from build123d import *

# Parameters (mm, degrees)
BOSS_EXTRUDE1_DEPTH = 1.6
SKETCH4_R           = 1.5
CUT_EXTRUDE1_DEPTH  = 1.6
SKETCH5_R           = 1.5
CUT_EXTRUDE2_DEPTH  = 1.6
SKETCH6_W           = 36.5
SKETCH6_H           = 3
CUT_EXTRUDE3_DEPTH  = 1.6
CUT_EXTRUDE4_DEPTH  = 1.6
CUT_EXTRUDE5_DEPTH  = 1.6
BOSS_EXTRUDE3_START = 1.6
SKETCH9_W           = 81.8
SKETCH9_H           = 2
BOSS_EXTRUDE3_DEPTH = 1


with BuildPart() as part:
    # Sketch2 → Boss-Extrude1 (new body)
    with BuildSketch(Plane.XY):
        Polygon((50, -51.75), (50, 4.25), (33.5, 51.75), (-33.5, 51.75), (-50, 4.25), (-50, -51.75), align=None)
    extrude(amount=BOSS_EXTRUDE1_DEPTH)

    # Sketch4 → Cut-Extrude1 (cut)
    with BuildSketch(Plane.XY.offset(1.6)):
        with Locations((-45.5, -48.75)):
            Circle(SKETCH4_R)
        with Locations((-45.5, -26.75)):
            Circle(SKETCH4_R)
        with Locations(Location((45.5, -26.75, 0), (0, 0, 180))):
            Circle(SKETCH4_R)
        with Locations(Location((45.5, -48.75, 0), (0, 0, 180))):
            Circle(SKETCH4_R)
    extrude(amount=-CUT_EXTRUDE1_DEPTH, mode=Mode.SUBTRACT)

    # Sketch5 → Cut-Extrude2 (cut)
    with BuildSketch(Plane.XY.offset(1.6)):
        with Locations((-18.25, 39.25)):
            Circle(SKETCH5_R)
        with Locations(Location((18.25, 39.25, 0), (0, 0, 180))):
            Circle(SKETCH5_R)
    extrude(amount=-CUT_EXTRUDE2_DEPTH, mode=Mode.SUBTRACT)

    # Sketch6 → Cut-Extrude3 (cut)
    with BuildSketch(Plane.XY.offset(1.6)):
        with Locations((0, 39.25)):
            Rectangle(SKETCH6_W, SKETCH6_H)
    extrude(amount=-CUT_EXTRUDE3_DEPTH, mode=Mode.SUBTRACT)

    # Sketch7 → Cut-Extrude4 (cut)
    with BuildSketch(Plane.XY):
        with BuildLine():
            Line((-33.55, -11.75), (33.55, -11.75))
            ThreePointArc((33.55, -11.75), (34.575304833, -11.325304833), (35, -10.3))
            Line((35, -10.3), (35, -10.2))
            ThreePointArc((35, -10.2), (34.575304833, -9.174695167), (33.55, -8.75))
            Line((33.55, -8.75), (-33.55, -8.75))
            ThreePointArc((-33.55, -8.75), (-34.575304833, -9.174695167), (-35, -10.2))
            Line((-35, -10.2), (-35, -10.3))
            ThreePointArc((-35, -10.3), (-34.575304833, -11.325304833), (-33.55, -11.75))
        make_face()
    extrude(amount=CUT_EXTRUDE4_DEPTH, mode=Mode.SUBTRACT)

    # Sketch8 → Cut-Extrude5 (cut)
    with BuildSketch(Plane.XY):
        with BuildLine():
            Line((-33.55, 11.25), (33.55, 11.25))
            ThreePointArc((33.55, 11.25), (34.575304833, 11.674695167), (35, 12.7))
            Line((35, 12.7), (35, 12.8))
            ThreePointArc((35, 12.8), (34.575304833, 13.825304833), (33.55, 14.25))
            Line((33.55, 14.25), (-33.55, 14.25))
            ThreePointArc((-33.55, 14.25), (-34.575304833, 13.825304833), (-35, 12.8))
            Line((-35, 12.8), (-35, 12.7))
            ThreePointArc((-35, 12.7), (-34.575304833, 11.674695167), (-33.55, 11.25))
        make_face()
    extrude(amount=CUT_EXTRUDE5_DEPTH, mode=Mode.SUBTRACT)

    # Sketch9 → Boss-Extrude3 (add)
    with BuildSketch(Plane.XY.offset(BOSS_EXTRUDE3_START)):
        Polygon((50, -23.75), (50, 4.25), (33.5, 51.75), (-33.5, 51.75), (-50, 4.25), (-50, -23.75), (-48, -23.75), (-48, 3.91252214), (-32.077507691, 49.75), (32.077507691, 49.75), (48, 3.91252214), (48, -23.75), align=None)
        with Locations((0, -50.75)):
            Rectangle(SKETCH9_W, SKETCH9_H)
    extrude(amount=BOSS_EXTRUDE3_DEPTH)


solid = part.part
For this review, take the finished solid that the model builds, in its own axes (mm). A direction names the side the tool comes from. Coordinates: 2 decimals unless noted, no trailing zeros. Write each loop counter-clockwise with the first axis right and the second up, starting at its lowest first coordinate (ties: lowest second). Pieces come first, ordered by that corner, then holes. Notation, with made-up numbers: (4, 25) -> (40, 25) arc R18 ccw to (40, 41) -> close; hole circle Ø11 at (-5, -27.75). An arc over 180 degrees is marked (long way). Write each question's results on one line, items separated by ' | '. Start each with the question number.
1) Consider section C-C (y = 26.5). Write out the cut boundary in (x, z), plus the area to 3 significant figures.
2) Insertion check: pin 1 (6 mm diameter, centred on x = -32, y = 36, fed in from +Z); pin 2 (2.5 mm diameter, centred on x = -45.5, y = -48.75, fed in from +Z). Each pin has a flat end and moves straight along its axis. Give the tip position at first contact, or say it passes through.
3) Consider section D-D (x = 45.5). Write out the cut boundary in (y, z).
4) Consider section A-A (z = 0.7). Give the number of separate pieces and of enclosed holes in the cut face, plus the area to 4 significant figures.
5) Consider section B-B (x = -24). Write out the cut boundary in (y, z).
6) Wall thickness on L1, parallel to Y at x = 16.5, z = 0.85; L2, parallel to Y at x = -23, z = 2.2; L3, parallel to Z at x = 20.5, y = 11: over which ranges is each line inside the solid? List them lowest first. Write a range as [from, to].
7) The part is to be moulded in two halves that separate along X. For faces 1 (the face through (0, 51.75, 1)), 2 (the face through (-41.634, 28.332, 1.282)), 3 (the face through (50, -24, 1)), 4 (the face through (46.69, -47.84, 0.81)), say which applies: +X half, -X half, draft (parallel to the pull), parting line (faces both ways), or undercut.
8) For faces 5 (the face through (-40.15, 26.51, 2.09)), 6 (the face through (-50, -23, 1)), list the 3-axis set-ups (+Z, -Z, +X, -X, +Y, -Y) from which the entire face can be reached by the end or side of a thin tool; tool diameter is ignored.
Geometry says:
1) outline: (-42.27, 0) -> (42.27, 0) -> (42.27, 2.6) -> (40.15, 2.6) -> (40.15, 1.6) -> (-40.15, 1.6) -> (-40.15, 2.6) -> (-42.27, 2.6) -> close | area: 140 mm^2
2) pin 1: z = 1.6 | pin 2: through
3) outline: (-51.75, 0) -> (-50.25, 0) -> (-50.25, 1.6) -> (-51.75, 1.6) -> close; (-47.25, 0) -> (-28.25, 0) -> (-28.25, 1.6) -> (-47.25, 1.6) -> close; (-25.25, 0) -> (17.2, 0) -> (17.2, 2.6) -> (11.11, 2.6) -> (11.11, 1.6) -> (-25.25, 1.6) -> close
4) separate pieces: 1 | enclosed holes: 7 | area: 9,005 mm^2
5) outline: (-51.75, 0) -> (-11.75, 0) -> (-11.75, 1.6) -> (-49.75, 1.6) -> (-49.75, 2.6) -> (-51.75, 2.6) -> close; (-8.75, 0) -> (11.25, 0) -> (11.25, 1.6) -> (-8.75, 1.6) -> close; (14.25, 0) -> (51.75, 0) -> (51.75, 2.6) -> (49.75, 2.6) -> (49.75, 1.6) -> (14.25, 1.6) -> close
6) L1: [-51.75, -11.75], [-8.75, 11.25], [14.25, 37.75], [40.75, 51.75] | L2: [-51.75, -49.75], [49.75, 51.75] | L3: [0, 1.6]
7) face 1: draft | face 2: -X half | face 3: +X half | face 4: undercut
8) face 5: +Z | face 6: +Z, -Z, -X, +Y, -Y
